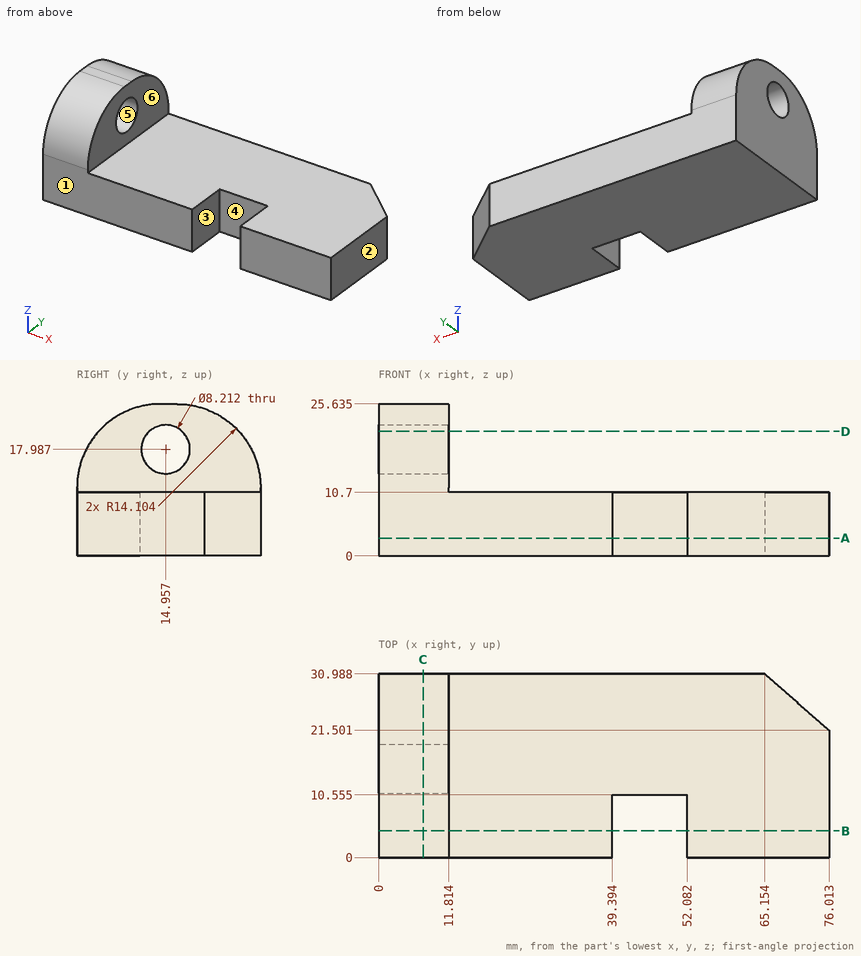
Could you check a few things on this drawing? It's one solid part, dimensions in mm from its lowest x, y, z. A direction names the side the tool comes from. Give positions to 0.01 mm unless a question says otherwise; leave off trailing zeros. Order: outer loops, then holes, each group sorted by start corner. A loop starts at its lowest first (then second) coordinate and runs counter-clockwise, first axis right, second up. Notation, with made-up numbers: (-36.5, -35) - (-7.5, -35) arc R6 ccw to (-7.5, -24) - close; hole circle Ø1 at (23, 59.25). An arc over 180 degrees is marked (long way). Answer as a JSON object with one key per item and string values. Group by question number.
Item 1: Which directions (+Z, -Z, +X, -X, +Y, -Y) give clear straight access to the entire face, cutting with the end or side of a thin tool? Please do the marked faces 4, 5 and 6.
Item 2: If we section it at B-B on y = 4.5: Please give me the cut outline in (x, z) (1 decimal).
Item 3: If we mould it in two halves opening along X, with no side actions, what happens to the marked faces 1, 2 and 3? For each: pulls with the +X half, pulls with the -X half, needs draft (parallel to the pull), parting line crosses it, or undercut.
Item 4: Please list where these lines run through material, in increasing order: probe 1 along X at (y, z) = (8, 8); probe 2 along X at (y, z) = (10, 10.75) (1 decimal); probe 3 along Z at (x, y) = (49, 22).
Item 5: If we section it at C-C on x = 7.5: Please give me the cut outline in (y, z) (1 decimal), and give its area (3 significant figures).
Item 6: For P1, Ø5, axis at y = 14.96, z = 17.99, coming from the -X side; P2, Ø10, axis at x = 49.5, y = 16, coming from the +Z side; P3, Ø4.5, axis at y = 8.5, z = 16.5, coming from the +X side, each with a flat end and sliding along its axis, tell me the tip position at first contact or that it passes through.
Item 7: If we section it at D-D on z = 21: Please give me the cut outline in (x, y) (1 decimal).
Item 8: If we section it at A-A on z = 3: Please give me the cut outline in (x, y) (1 decimal).
Result set:
{
 "1": {"face 4": "+Z, -Z, -Y", "face 5": "+X, -X", "face 6": "+Z, +X, +Y, -Y"},
 "2": {"outline": "(0, 0) - (39.4, 0) - (39.4, 10.7) - (11.8, 10.7) - (11.8, 21.9) - (0, 21.9) - close; (52.1, 0) - (76, 0) - (76, 10.7) - (52.1, 10.7) - close"},
 "3": {"face 1": "needs draft", "face 2": "pulls with the +X half", "face 3": "undercut"},
 "4": {"probe 1": "0 to 39.39, 52.08 to 76.01", "probe 2": "0 to 11.8", "probe 3": "0 to 10.7"},
 "5": {"outline": "(0, 0) - (31, 0) - (31, 11.5) arc R14.1 ccw to (16.9, 25.6) - (14.1, 25.6) arc R14.1 ccw to (0, 11.5) - close; hole circle Ø8.2 at (15, 18)", "area": "656 mm²"},
 "6": {"P1": "through", "P2": "z = 10.7", "P3": "x = 11.81"},
 "7": {"outline": "(0, 3.7) - (11.8, 3.7) - (11.8, 12.2) - (0, 12.2) - close; (0, 17.7) - (11.8, 17.7) - (11.8, 27.3) - (0, 27.3) - close"},
 "8": {"outline": "(0, 0) - (39.4, 0) - (39.4, 10.6) - (52.1, 10.6) - (52.1, 0) - (76, 0) - (76, 21.5) - (65.2, 31) - (0, 31) - close"}
}
